```python
from build123d import *

# Parameters (mm, degrees)
SKETCH2_R             = 37.5
SKETCH2_R_2           = 2.5
BOSS_EXTRUDE1_DEPTH   = 15
SKETCH3_R             = 4.5
CUT_EXTRUDE1_DEPTH    = 6
M6X1_0_TAPPED_HOLE1_D = 5


with BuildPart() as part:
    # Sketch2 → Boss-Extrude1 (new body)
    with BuildSketch(Plane(origin=(0, 0, 0), x_dir=(1, 0, 0), z_dir=(0, 1, 0))):
        Circle(SKETCH2_R)
        with Locations((-18.679244128, 19.315419379)):
            Circle(SKETCH2_R_2, mode=Mode.SUBTRACT)
        with Locations((19.315419379, 18.679244128)):
            Circle(SKETCH2_R_2, mode=Mode.SUBTRACT)
        with Locations((18.679244128, -19.315419379)):
            Circle(SKETCH2_R_2, mode=Mode.SUBTRACT)
        with Locations((-19.315419379, -18.679244128)):
            Circle(SKETCH2_R_2, mode=Mode.SUBTRACT)
    extrude(amount=BOSS_EXTRUDE1_DEPTH)

    # Sketch3 → Cut-Extrude1 (cut)
    with BuildSketch(Plane(origin=(0, 15, 0), x_dir=(1, 0, 0), z_dir=(0, 1, 0))):
        with Locations((-18.679244128, 19.315419379)):
            Circle(SKETCH3_R)
        with Locations((19.315419379, 18.679244128)):
            Circle(SKETCH3_R)
        with Locations((18.679244128, -19.315419379)):
            Circle(SKETCH3_R)
        with Locations((-19.315419379, -18.679244128)):
            Circle(SKETCH3_R)
    extrude(amount=-CUT_EXTRUDE1_DEPTH, mode=Mode.SUBTRACT)

    # M6x1.0 Tapped Hole1 (through all)
    with Locations(Plane(origin=(0, 15, -31), x_dir=(0, 0, 1), z_dir=(0, 1, 0))):
        with Locations((0, 0), (15.5, 26.846787517), (46.5, 26.846787517), (62, 0), (46.5, -26.846787517), (15.5, -26.846787517)):
            Hole(M6X1_0_TAPPED_HOLE1_D / 2)


solid = part.part
```
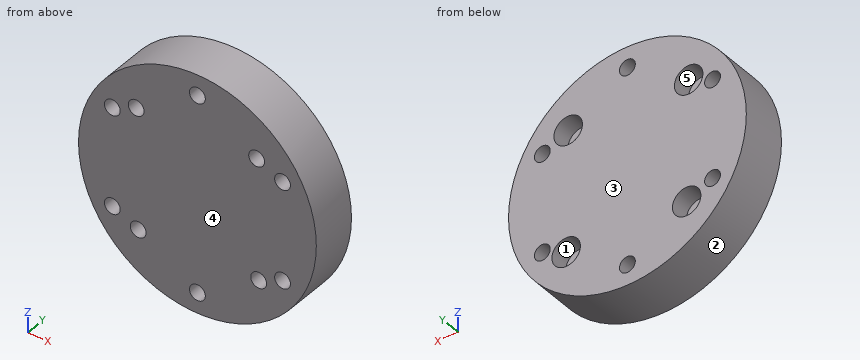
Read the model definition and answer for the solid it produces. Units are mm, in the model's axes. Face numbers are marked on the shaded views. A direction names the side the tool comes from. Coordinates: 2 decimals unless noted, no trailing zeros. Write each loop counter-clockwise with the first axis right and the second up, starting at its lowest first coordinate (ties: lowest second). Pieces come first, ordered by that corner, then holes. Notation, with made-up numbers: (-4.5, 61.25) - (1.5, 61.25) arc R5 ccw to (1.5, 68.25) - close; hole circle Ø4 at (64.5, -33). An arc over 180 degrees is marked (long way). Answer as a JSON object with one key per item and string values. Group by question number.
1. The mould has two halves that part along Z. Classify the marked faces 1, 2 and 3: +Z half, -Z half, draft (parallel to the pull), parting line (faces both ways), or undercut.
2. Consider L1, parallel to X at y = 6, z = 16; L2, parallel to Z at x = -29, y = 6.5; L3, parallel to Z at x = 20.5, y = 14.25. Determine where each line is inside the solid, lowest interval first. Write a range as [from, to].
3. A cutting plane is placed at A-A (x = 0). Determine the outline of the cut face in (y, z), plus the area to 3 significant figures.
4. A cutting plane is placed at C-C (z = 31). Determine the outline of the cut face in (x, y), plus the area to 3 significant figures.
5. Each of these flat-tipped pins is pushed along its axis until it touches: P1, Ø6.5, axis at x = -19.32, z = 18.68, coming from the +Y side; P2, Ø2, axis at y = 13, z = -26, coming from the -X side. Where does it stop, or does it pass through?
6. A cutting plane is placed at B-B (y = 4.5). Give the number of separate pieces and of enclosed holes in the cut face, plus the area to 3 significant figures.
7. Which of the six approach directions +Z, -Z, +X, -X, +Y, -Y give full straight-line access (tool end or side, diameter ignored) to the marked faces 4 and 5?
Worked out:
{
 "1": {"face 1": "undercut", "face 2": "parting line", "face 3": "draft"},
 "2": {"L1": "x = [-33.92, -29.3], [-24.4, 24.4], [29.3, 33.92]", "L2": "z = [-23.77, -16.77], [-14.23, 14.23], [16.77, 23.77]", "L3": "z = [-31.4, -23.02], [-14.34, 15.2], [23.43, 31.4]"},
 "3": {"outline": "(0, -37.5) - (15, -37.5) - (15, -33.5) - (0, -33.5) - close; (0, -28.5) - (15, -28.5) - (15, 28.5) - (0, 28.5) - close; (0, 33.5) - (15, 33.5) - (15, 37.5) - (0, 37.5) - close", "area": "975 mm²"},
 "4": {"outline": "(-21.1, 0) - (-2.5, 0) - (-2.5, 15) - (-21.1, 15) - close; (2.5, 0) - (21.1, 0) - (21.1, 15) - (2.5, 15) - close", "area": "558 mm²"},
 "5": {"P1": "stops at y = 9", "P2": "stops at x = -27.95"},
 "6": {"separate pieces": "1", "enclosed holes": "10", "area": "4,220 mm²"},
 "7": {"face 4": "+Z, -Z, +X, -X, -Y", "face 5": "+Y"}
}
